```python
from build123d import *

# Parameters (mm, degrees)
SKETCH1_W            = 35
SKETCH1_H            = 30
SKETCH1_R            = 2.1
BOSS_EXTRUDE1_DEPTH  = 5
SKETCH2_W            = 30
SKETCH2_H            = 17
BOSS_EXTRUDE2_DEPTH  = 5
BOSS_EXTRUDE3_START  = -28
BOSS_EXTRUDE3_DEPTH  = 37
CUT_EXTRUDE1_REACH   = 66.542
CUT_EXTRUDE1_START   = -4.5
SKETCH5_W            = 36
SKETCH5_H            = 12.013565991
SKETCH6_W            = 2.1
SKETCH6_H            = 35.25
CUT_EXTRUDE2_DEPTH   = 5
SKETCH9_W            = 9.9
SKETCH9_H            = 8
BOSS_EXTRUDE5_DEPTH  = 5
SKETCH10_W           = 0.7
SKETCH10_H           = 46
CUT_EXTRUDE4_DEPTH   = 5
CUT_EXTRUDE5_REACH   = 68.83
SKETCH7_R            = 2.1
SKETCH11_W           = 17.6
SKETCH11_H           = 20
SKETCH11_W_2         = 15
SKETCH11_H_2         = 2
BOSS_EXTRUDE6_DEPTH  = 11
SKETCH12_W           = 15
SKETCH12_H           = 24
BOSS_EXTRUDE8_DEPTH  = 2
SKETCH13_W           = 2
SKETCH13_H           = 20
BOSS_EXTRUDE9_DEPTH  = 11
SKETCH14_W           = 17.6
SKETCH14_H           = 20
BOSS_EXTRUDE10_DEPTH = 2
CUT_EXTRUDE6_START   = -36
SKETCH15_R           = 2.1
CUT_EXTRUDE6_DEPTH   = 36
SKETCH16_R           = 4
SKETCH16_R_2         = 4.5
CUT_EXTRUDE7_DEPTH   = 8
BOSS_EXTRUDE11_START = -2
SKETCH17_R           = 3.3
SKETCH17_R_2         = 2.1
BOSS_EXTRUDE11_DEPTH = 1
BOSS_EXTRUDE12_START = -12
SKETCH17_2_R         = 3.3
SKETCH17_2_R_2       = 2.1
BOSS_EXTRUDE12_DEPTH = 1
BOSS_EXTRUDE13_START = -2
SKETCH18_R           = 3.3
SKETCH18_R_2         = 2.1
BOSS_EXTRUDE13_DEPTH = 1
BOSS_EXTRUDE14_START = -12
SKETCH18_2_R         = 3.3
SKETCH18_2_R_2       = 2.1
BOSS_EXTRUDE14_DEPTH = 1
SKETCH19_R           = 1.55
CUT_EXTRUDE8_DEPTH   = 95.781405877


with BuildPart() as part:
    # Sketch1 → Boss-Extrude1 (new body)
    with BuildSketch(Plane(origin=(0, 0, 0), x_dir=(1, 0, 0), z_dir=(0, 1, 0))):
        Rectangle(SKETCH1_W, SKETCH1_H)
        with Locations(Location((12, 9, 0), (0, 0, 270))):
            Circle(SKETCH1_R, mode=Mode.SUBTRACT)
        with Locations(Location((12, -9, 0), (0, 0, 90))):
            Circle(SKETCH1_R, mode=Mode.SUBTRACT)
        with Locations(Location((-12, -9, 0), (0, 0, 270))):
            Circle(SKETCH1_R, mode=Mode.SUBTRACT)
        with Locations(Location((-12, 9, 0), (0, 0, 90))):
            Circle(SKETCH1_R, mode=Mode.SUBTRACT)
    extrude(amount=BOSS_EXTRUDE1_DEPTH)

    # Sketch2 → Boss-Extrude2 (add)
    with BuildSketch(Plane.ZY.offset(17.5)):
        with Locations((0, -3.5)):
            Rectangle(SKETCH2_W, SKETCH2_H)
    extrude(amount=BOSS_EXTRUDE2_DEPTH)

    # Sketch3 → Boss-Extrude3 (add)
    with BuildSketch(Plane(origin=(17.5, 0, 0), x_dir=(0, 0, -1), z_dir=(1, 0, 0)).offset(BOSS_EXTRUDE3_START)):
        with BuildLine():
            Line((-41, 0), (41, 0))
            Line((41, 0), (41, -12))
            Line((41, -12), (37.43, -12))
            Line((37.43, -12), (37.43, -18))
            Line((37.43, -18), (35.03, -18))
            Line((35.03, -18), (35.03, -12))
            Line((35.03, -12), (35.03, -10.095119046))
            ThreePointArc((35.03, -10.095119046), (34.83, -1.9), (34.63, -10.095119046))
            Line((34.63, -10.095119046), (34.63, -12))
            Line((34.63, -12), (34.63, -18))
            Line((34.63, -18), (32.23, -18))
            Line((32.23, -18), (32.23, -12))
            Line((32.23, -12), (-32.23, -12))
            Line((-32.23, -12), (-32.23, -18))
            Line((-32.23, -18), (-34.63, -18))
            Line((-34.63, -18), (-34.63, -12))
            Line((-34.63, -12), (-34.63, -10.095119046))
            ThreePointArc((-34.63, -10.095119046), (-34.83, -1.9), (-35.03, -10.095119046))
            Line((-35.03, -10.095119046), (-35.03, -12))
            Line((-35.03, -12), (-35.03, -18))
            Line((-35.03, -18), (-37.43, -18))
            Line((-37.43, -18), (-37.43, -12))
            Line((-37.43, -12), (-41, -12))
            Line((-41, -12), (-41, 0))
        make_face()
    extrude(amount=-BOSS_EXTRUDE3_DEPTH)

    # Sketch5 → Cut-Extrude1 (cut, up to next)
    with BuildSketch(Plane.ZY.offset(22.5).offset(CUT_EXTRUDE1_START), mode=Mode.PRIVATE) as cut_extrude1_sk1:
        with Locations((0, -5.993217004)):
            Rectangle(SKETCH5_W, SKETCH5_H)
    cut_extrude1_tool1 = extrude(cut_extrude1_sk1.sketch, amount=-CUT_EXTRUDE1_REACH, mode=Mode.PRIVATE) & part.part
    add(cut_extrude1_tool1.solids().sort_by_distance((-18, -5.993217, 0))[0], mode=Mode.SUBTRACT)

    # Sketch6 → Cut-Extrude2 (cut)
    with BuildSketch(Plane(origin=(0, 5, 0), x_dir=(1, 0, 0), z_dir=(0, 1, 0))):
        with Locations((-21.45, -2.625)):
            Rectangle(SKETCH6_W, SKETCH6_H)
    extrude(amount=-CUT_EXTRUDE2_DEPTH, mode=Mode.SUBTRACT)

    # Sketch9 → Boss-Extrude5 (add)
    with BuildSketch(Plane(origin=(0, 0, 0), x_dir=(1, 0, 0), z_dir=(0, 1, 0))):
        with Locations((-15.45, 19)):
            Rectangle(SKETCH9_W, SKETCH9_H)
        with Locations((-15.45, -19)):
            Rectangle(SKETCH9_W, SKETCH9_H)
    extrude(amount=BOSS_EXTRUDE5_DEPTH)

    # Sketch10 → Cut-Extrude4 (cut)
    with BuildSketch(Plane(origin=(0, 5, 0), x_dir=(1, 0, 0), z_dir=(0, 1, 0))):
        with Locations((-20.05, 0)):
            Rectangle(SKETCH10_W, SKETCH10_H)
    extrude(amount=-CUT_EXTRUDE4_DEPTH, mode=Mode.SUBTRACT)

    # Sketch7 → Cut-Extrude5 (cut, up to next)
    with BuildSketch(Plane(origin=(0, 5, 0), x_dir=(1, 0, 0), z_dir=(0, 1, 0)), mode=Mode.PRIVATE) as cut_extrude5_sk1:
        with Locations(Location((-41.9, -20.25, 0), (0, 0, 270))):
            Circle(SKETCH7_R)
    cut_extrude5_tool1 = extrude(cut_extrude5_sk1.sketch, amount=-CUT_EXTRUDE5_REACH, mode=Mode.PRIVATE) & part.part
    # Sketch7 → Cut-Extrude5 (cut, up to next)
    with BuildSketch(Plane(origin=(0, 5, 0), x_dir=(1, 0, 0), z_dir=(0, 1, 0)), mode=Mode.PRIVATE) as cut_extrude5_sk2:
        with Locations(Location((-29.9, 20.25, 0), (0, 0, 270))):
            Circle(SKETCH7_R)
    cut_extrude5_tool2 = extrude(cut_extrude5_sk2.sketch, amount=-CUT_EXTRUDE5_REACH, mode=Mode.PRIVATE) & part.part
    add(cut_extrude5_tool1.solids().sort_by_distance((-41.9, 5, 20.25))[0], mode=Mode.SUBTRACT)
    add(cut_extrude5_tool2.solids().sort_by_distance((-29.9, 5, -20.25))[0], mode=Mode.SUBTRACT)

    # Sketch11 → Boss-Extrude6 (add)
    with BuildSketch(Plane(origin=(0, 0, 0), x_dir=(1, 0, 0), z_dir=(0, 1, 0))):
        with Locations((-38.7, -20.25)):
            Rectangle(SKETCH11_W, SKETCH11_H)
        with Locations((-32.4, 31.25)):
            Rectangle(SKETCH11_W_2, SKETCH11_H_2)
        with Locations((-32.4, 9.25)):
            Rectangle(SKETCH11_W_2, SKETCH11_H_2)
    extrude(amount=BOSS_EXTRUDE6_DEPTH)

    # Sketch12 → Boss-Extrude8 (add)
    with BuildSketch(Plane(origin=(0, 11, 0), x_dir=(1, 0, 0), z_dir=(0, 1, 0))):
        with Locations((-32.4, 20.25)):
            Rectangle(SKETCH12_W, SKETCH12_H)
    extrude(amount=BOSS_EXTRUDE8_DEPTH)

    # Sketch13 → Boss-Extrude9 (add)
    with BuildSketch(Plane(origin=(0, 11, 0), x_dir=(1, 0, 0), z_dir=(0, 1, 0))):
        with Locations((-30.9, -20.25)):
            Rectangle(SKETCH13_W, SKETCH13_H)
    extrude(amount=BOSS_EXTRUDE9_DEPTH)

    # Sketch14 → Boss-Extrude10 (add)
    with BuildSketch(Plane(origin=(0, 22, 0), x_dir=(1, 0, 0), z_dir=(0, 1, 0))):
        with Locations((-38.7, -20.25)):
            Rectangle(SKETCH14_W, SKETCH14_H)
    extrude(amount=BOSS_EXTRUDE10_DEPTH)

    # Sketch15 → Cut-Extrude6 (cut)
    with BuildSketch(Plane.XZ.offset(12).offset(CUT_EXTRUDE6_START)):
        with Locations(Location((-29.9, -20.25, 0), (0, 0, 90))):
            Circle(SKETCH15_R)
        with Locations(Location((-41.9, 20.25, 0), (0, 0, 90))):
            Circle(SKETCH15_R)
    extrude(amount=CUT_EXTRUDE6_DEPTH, mode=Mode.SUBTRACT)

    # Sketch16 → Cut-Extrude7 (cut)
    with BuildSketch(Plane.XZ.offset(12)):
        with Locations(Location((-41.9, 20.25, 0), (0, 0, 270))):
            Circle(SKETCH16_R)
        with Locations(Location((-29.9, -20.25, 0), (0, 0, 270))):
            Circle(SKETCH16_R_2)
    extrude(amount=-CUT_EXTRUDE7_DEPTH, mode=Mode.SUBTRACT)

    # Sketch17 → Boss-Extrude11 (add)
    with BuildSketch(Plane(origin=(0, 24, 0), x_dir=(1, 0, 0), z_dir=(0, 1, 0)).offset(BOSS_EXTRUDE11_START)):
        with Locations(Location((-41.9, -20.25, 0), (0, 0, 270))):
            Circle(SKETCH17_R)
        with Locations(Location((-41.9, -20.25, 0), (0, 0, 90))):
            Circle(SKETCH17_R_2, mode=Mode.SUBTRACT)
    extrude(amount=-BOSS_EXTRUDE11_DEPTH)

    # Sketch17<2> → Boss-Extrude12 (add)
    with BuildSketch(Plane(origin=(0, 24, 0), x_dir=(1, 0, 0), z_dir=(0, 1, 0)).offset(BOSS_EXTRUDE12_START)):
        with Locations(Location((-41.9, -20.25, 0), (0, 0, 270))):
            Circle(SKETCH17_2_R)
        with Locations(Location((-41.9, -20.25, 0), (0, 0, 90))):
            Circle(SKETCH17_2_R_2, mode=Mode.SUBTRACT)
    extrude(amount=-BOSS_EXTRUDE12_DEPTH)

    # Sketch18 → Boss-Extrude13 (add)
    with BuildSketch(Plane(origin=(0, 13, 0), x_dir=(1, 0, 0), z_dir=(0, 1, 0)).offset(BOSS_EXTRUDE13_START)):
        with Locations(Location((-29.9, 20.25, 0), (0, 0, 270))):
            Circle(SKETCH18_R)
        with Locations(Location((-29.9, 20.25, 0), (0, 0, 90))):
            Circle(SKETCH18_R_2, mode=Mode.SUBTRACT)
    extrude(amount=-BOSS_EXTRUDE13_DEPTH)

    # Sketch18<2> → Boss-Extrude14 (add)
    with BuildSketch(Plane(origin=(0, 13, 0), x_dir=(1, 0, 0), z_dir=(0, 1, 0)).offset(BOSS_EXTRUDE14_START)):
        with Locations(Location((-29.9, 20.25, 0), (0, 0, 270))):
            Circle(SKETCH18_2_R)
        with Locations(Location((-29.9, 20.25, 0), (0, 0, 90))):
            Circle(SKETCH18_2_R_2, mode=Mode.SUBTRACT)
    extrude(amount=-BOSS_EXTRUDE14_DEPTH)

    # Sketch19 → Cut-Extrude8 (cut, through all)
    with BuildSketch(Plane.XY.offset(37.43)):
        with Locations((-40.5, -15)):
            Circle(SKETCH19_R)
        with Locations((-17.5, -15)):
            Circle(SKETCH19_R)
    extrude(amount=-CUT_EXTRUDE8_DEPTH, mode=Mode.SUBTRACT)


solid = part.part
```
Geometry check sheet. Reference: the model listing, model coordinates, mm. A direction names the side the tool comes from. Coordinates: 2 decimals unless noted, no trailing zeros. Order: outer loops, then holes, each group sorted by start corner. A loop starts at its lowest first (then second) coordinate and runs counter-clockwise, first axis right, second up. Notation, with made-up numbers: M 89,8.5 L 123,8.5 A15 ccw 123,29.5 Z; hole C 65.25,-25 d4. An arc over 180 degrees is marked long. Answer as a JSON object with one key per item and string values.
Q1. Release check for a two-part mould opening along Y. For faces 6 (the cylindrical face through (-39.1, 21.5, 22)), 7 (the flat face through (-38, 22, 20)), 8 (the flat face through (-15, 2, -23)), 9 (the flat face through (-39, 24, 20)) record: released by +Y, released by -Y, zero draft, split by the parting line, or undercut.
Results are:
{"face 6": "undercut", "face 7": "undercut", "face 8": "zero draft", "face 9": "released by +Y"}
Q2. Tool access check on faces 1 (the flat face through (-33, 5, -30.25)), 2 (the flat face through (-33, 5, -10.25)), 3 (the cylindrical face through (-26.63, 0.51, -20.68)), 4 (the cylindrical face through (-44.334, -8.056, 23.424)), 5 (the flat face through (-18, -6, 0)). Record the directions out of +Z, -Z, +X, -X, +Y, -Y that give a thin tool (end or side, any length) a straight path to the whole face; none if there is none.
Results are:
{"face 1": "+X, -X", "face 2": "-X", "face 3": "none", "face 4": "-Y", "face 5": "+X, -Y"}
Q3. Scan lines: line 1 (Z direction, x = -24, y = -10.5); line 2 (Y direction, x = -40.5, z = -36.25); line 3 (Z direction, x = -12, y = 2). Record each from-to range of solid material in increasing order.
Results are:
{"line 1": "z = -41 to -35.03, -34.63 to 34.63, 35.03 to 41", "line 2": "y = -18 to -16.55, -13.45 to -9.85, -2.15 to 0", "line 3": "z = -23 to -11.1, -6.9 to 6.9, 11.1 to 23"}
Q4. Cross-section at B-B on z = -13. Record the cut outline in (x, y), and give its area (3 significant figures).
Results are:
{"outline": "M -47.5,-12 L -18,-12 L -18,0.01 L 17.5,0.01 L 17.5,5 L -19.7,5 L -19.7,0 L -47.5,0 Z; M -39.9,11 L -24.9,11 L -24.9,13 L -39.9,13 Z", "area": "570 mm²"}
Q5. Cross-section at C-C on y = 9. Record the cut outline in (x, z).
Results are:
{"outline": "M -47.5,10.25 L -29.9,10.25 L -29.9,30.25 L -47.5,30.25 Z; M -39.9,-32.25 L -24.9,-32.25 L -24.9,-30.25 L -39.9,-30.25 Z; M -39.9,-10.25 L -24.9,-10.25 L -24.9,-8.25 L -39.9,-8.25 Z; hole C -41.9,20.25 d4.2"}
Q6. Depth check by flat-ended pin: pin 1 Ø18.5 at (x, z) = (-23.5, -2.5) entering from +Y; pin 2 Ø12 at (x, z) = (9, -16.5) entering from +Y; pin 3 Ø11 at (x, z) = (-33, 1) entering from -Y; pin 4 Ø2.5 at (x, y) = (-40.5, -15) entering from -Z. Enter the tip coordinate at first touch or a pass-through.
Results are:
{"pin 1": "stops at y = 13", "pin 2": "stops at y = 5", "pin 3": "stops at y = -12", "pin 4": "passes through"}
Q7. Cross-section at D-D on x = 12. Record the cut outline in (y, z).
Results are:
{"outline": "M 0.01,-15 L 5,-15 L 5,-11.1 L 0.01,-11.1 Z; M 0.01,-6.9 L 5,-6.9 L 5,6.9 L 0.01,6.9 Z; M 0.01,11.1 L 5,11.1 L 5,15 L 0.01,15 Z"}
Q8. Cross-section at A-A on y = 2. Give the number of separate pieces and of enclosed holes in the cut face, and give its area (3 significant figures).
Results are:
{"separate pieces": "4", "enclosed holes": "5", "area": "1,610 mm²"}
